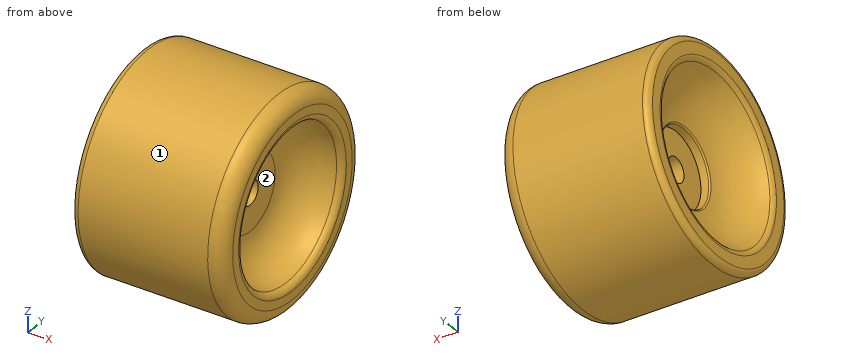
```python
from build123d import *


with BuildPart() as part:
    # Sketch1 → Revolve1 (revolve)
    with BuildSketch(Plane(origin=(0, 0, 0), x_dir=(-1, 0, 0), z_dir=(0, 0, -1)), mode=Mode.PRIVATE) as revolve1_sk:
        with BuildLine():
            Line((0, 4), (22, 4))
            Line((22, 4), (22, 12.5))
            Line((22, 12.5), (24.562401465, 12.5))
            ThreePointArc((24.562401465, 12.5), (24.889670699, 12.62198565), (25.057251332, 12.928420605))
            ThreePointArc((25.057251332, 12.928420605), (28.336858489, 21.346867264), (34.986476907, 27.463127736))
            ThreePointArc((34.986476907, 27.463127736), (35.728142618, 28.19617719), (36, 29.20291603))
            Line((36, 29.20291603), (36, 33))
            ThreePointArc((36, 33), (35.414213562, 34.414213562), (34, 35))
            Line((34, 35), (-9, 35))
            ThreePointArc((-9, 35), (-12.535533906, 33.535533906), (-14, 30))
            Line((-14, 30), (-14, 27.068802284))
            ThreePointArc((-14, 27.068802284), (-13.442084631, 25.683020225), (-12.079608083, 25.070387274))
            ThreePointArc((-12.079608083, 25.070387274), (-3.509387298, 21.216816616), (0, 12.5))
            Line((0, 12.5), (0, 4))
        make_face()
    revolve(revolve1_sk.sketch.rotate(Axis((14.002105865, 0, 0), (-1, 0, 0)), 270), axis=Axis((14.002105865, 0, 0), (-1, 0, 0)))


solid = part.part
```
Model file for the job. Use its own axes, mm. Face numbers are marked on the shaded views. Round coordinates to 2 decimals unless told otherwise and drop trailing zeros. Order: outer loops, then holes, each group sorted by start corner. A loop starts at its lowest first (then second) coordinate and runs counter-clockwise, first axis right, second up. Notation, with made-up numbers: (-34, 66.5) -> (-22, 66.5) arc R13 ccw to (-22, 75.5) -> close; hole circle Ø9 at (8, 53). An arc over 180 degrees is marked (long way). Use one line per item in the form item = value.
Item 1: Flat gauge pins, fed straight in: pin 1 Ø20 at (y, z) = (-4.5, 0.5) entering from +X; pin 2 Ø5 at (x, z) = (-14, 9.5) entering from -Y; pin 3 Ø12 at (x, z) = (-25, 22.5) entering from -Y. Where does each tip first touch, or does it go through?
Returned:
pin_1 = 0.16
pin_2 = -34.29
pin_3 = -30.87
Item 2: Cut at A-A, the plane x = -17.5. Write the cut outline in (y, z).
Returned:
outline = circle Ø70 at (0, 0); hole circle Ø8 at (0, 0)
Item 3: Pull direction Y, two halves, no side cores. Call the marked faces 1 and 2: released by +Y, released by -Y, zero draft, split by the parting line, or undercut.
Returned:
face_1 = split by the parting line
face_2 = undercut
Item 4: Drill centre lines: line 1 (Y direction, x = -6.75, z = 0); line 2 (Y direction, x = -22.8, z = 0); line 3 (X direction, y = 3, z = -4.5). Where is each one in solid material? Low to high.
Returned:
line_1 = -35 to -4, 4 to 35
line_2 = -35 to -12.5, 12.5 to 35
line_3 = -22 to 0
